Geometry: final body of the model. Coordinates: model frame, mm. A direction names the side the tool comes from. Give positions to 0.01 mm unless a question says otherwise; leave off trailing zeros. Write each loop counter-clockwise with the first axis right and the second up, starting at its lowest first coordinate (ties: lowest second). Pieces come first, ordered by that corner, then holes. Notation, with made-up numbers: (26.5, 38) -> (58.5, 38) arc R25 cw to (58.5, 56) -> close; hole circle Ø2 at (88.5, 35). An arc over 180 degrees is marked (long way). Answer in a Markdown table with one row per item. Add a question column.
Item 1: Section query A-A on y = -13.75. State how many separate pieces and enclosed holes the cut face has, plus the area to 3 significant figures.
Item 2: Access query for faces 1 (the flat face through (15.8, -10.8, 92.1)), 2 (the flat face through (-9.5, -16, 88)), 3 (the flat face through (16.507, 18.048, 38.711)). Directions: +Z, -Z, +X, -X, +Y, -Y. A direction counts if a zero-diameter tool reaches every point of the face in a straight line with its end or side. Return the directions, or none.
Item 3: Draft query along Z for faces 4 (the flat face through (-18.48, -3.58, 29.11)), 5 (the flat face through (13, -18, 12)), 6 (the flat face through (27, 0, 45)). Return one class per face: +Z half, -Z half, draft (parallel to the pull), parting line (faces both ways), or undercut.
Item 4: Material intervals for probe 1 along Y at (x, z) = (13, 4.6); probe 2 along Z at (x, y) = (17.5, -17); probe 3 along Z at (x, y) = (24.25, 13.75), sorted ascending. Write a range as from..to.
Item 5: Section query C-C on x = 22. Output: boundary loops of the cut face in (y, z).
Item 6: Section query D-D on z = 48.5. Output: boundary loops of the cut face in (x, y), plus the area to 3 significant figures.
```python
from build123d import *

# Parameters (mm, degrees)
SKETCH_W            = 54
SKETCH_H            = 44
PAD_DEPTH           = 92.5
SKETCH001_W         = 32
SKETCH001_H         = 44
POCKET_DEPTH        = 86.5
SKETCH002_R         = 2.25
HOLE_DEPTH          = 50
HOLE001_DEPTH       = 50
SKETCH003_R         = 1
HOLE002_DEPTH       = 12
HOLE003_D           = 3.5
HOLE003_DEPTH       = 25
HOLE003_CBORE_D     = 6
HOLE003_CBORE_DEPTH = 6
HOLE003_TIPS_R      = 1.75
POCKET001_DEPTH     = 4
POCKET002_DEPTH     = 4
CHAMFER_SIZE        = 1
SKETCH007_W         = 5
SKETCH007_H         = 8.5
POCKET003_DEPTH     = 13


with BuildPart() as part:
    # Sketch → Pad (new body)
    with BuildSketch(Plane.XY):
        Rectangle(SKETCH_W, SKETCH_H)
    extrude(amount=PAD_DEPTH)

    # Sketch001 (on Face6 of Pad) → Pocket (cut)
    with BuildSketch(Plane.XY.offset(92.5)):
        with Locations((0, 11)):
            Rectangle(SKETCH001_W, SKETCH001_H)
    extrude(amount=-POCKET_DEPTH, mode=Mode.SUBTRACT)

    # Sketch002 → Hole (cut)
    with BuildSketch(Plane.YZ):
        with Locations((0, 41)):
            Circle(SKETCH002_R)
        with Locations((13.75, 41)):
            Circle(SKETCH002_R)
        with Locations((0, 54.75)):
            Circle(SKETCH002_R)
        with Locations((0, 27.25)):
            Circle(SKETCH002_R)
        with Locations((-13.75, 41)):
            Circle(SKETCH002_R)
    extrude(amount=-HOLE_DEPTH, mode=Mode.SUBTRACT)

    # Sketch002 → Hole001 (cut)
    with BuildSketch(Plane.YZ):
        with Locations((0, 41)):
            Circle(SKETCH002_R)
        with Locations((13.75, 41)):
            Circle(SKETCH002_R)
        with Locations((0, 54.75)):
            Circle(SKETCH002_R)
        with Locations((0, 27.25)):
            Circle(SKETCH002_R)
        with Locations((-13.75, 41)):
            Circle(SKETCH002_R)
    extrude(amount=HOLE001_DEPTH, mode=Mode.SUBTRACT)

    # Sketch003 → Hole002 (cut)
    with BuildSketch(Plane.XY):
        with Locations((-13, 18.5)):
            Circle(SKETCH003_R)
        with Locations((13, 18.5)):
            Circle(SKETCH003_R)
        with Locations((13, -18.5)):
            Circle(SKETCH003_R)
        with Locations((-13, -18.5)):
            Circle(SKETCH003_R)
    extrude(amount=HOLE002_DEPTH, mode=Mode.SUBTRACT)

    # Hole003
    with Locations(Plane.XZ.offset(22)):
        with Locations((-11.5, 88), (11.5, 88), (11.5, 55), (-11.5, 55)):
            CounterBoreHole(HOLE003_D / 2, HOLE003_CBORE_D / 2, HOLE003_CBORE_DEPTH, depth=HOLE003_DEPTH)

    # Hole003 tips → Hole003 tip 1 section 0
    with BuildSketch(Plane.XZ.offset(-3), mode=Mode.PRIVATE) as hole003_tip_1_s0:
        with Locations((-11.5, 88)):
            Circle(HOLE003_TIPS_R)
    loft([hole003_tip_1_s0.sketch, Vertex(-11.5, 4.051506, 88)], mode=Mode.SUBTRACT)

    # Hole003 tips → Hole003 tip 2 section 0
    with BuildSketch(Plane.XZ.offset(-3), mode=Mode.PRIVATE) as hole003_tip_2_s0:
        with Locations((11.5, 88)):
            Circle(HOLE003_TIPS_R)
    loft([hole003_tip_2_s0.sketch, Vertex(11.5, 4.051506, 88)], mode=Mode.SUBTRACT)

    # Hole003 tips → Hole003 tip 3 section 0
    with BuildSketch(Plane.XZ.offset(-3), mode=Mode.PRIVATE) as hole003_tip_3_s0:
        with Locations((11.5, 55)):
            Circle(HOLE003_TIPS_R)
    loft([hole003_tip_3_s0.sketch, Vertex(11.5, 4.051506, 55)], mode=Mode.SUBTRACT)

    # Hole003 tips → Hole003 tip 4 section 0
    with BuildSketch(Plane.XZ.offset(-3), mode=Mode.PRIVATE) as hole003_tip_4_s0:
        with Locations((-11.5, 55)):
            Circle(HOLE003_TIPS_R)
    loft([hole003_tip_4_s0.sketch, Vertex(-11.5, 4.051506, 55)], mode=Mode.SUBTRACT)

    # Sketch005 → Pocket001 (cut)
    with BuildSketch(Plane(origin=(16, 0, 0), x_dir=(0, -1, 0), z_dir=(-1, 0, 0))):
        Polygon((2.4, 50.843078), (4.8, 55), (2.4, 59.156922), (-2.4, 59.156922), (-4.8, 55), (-2.4, 50.843078), align=None)
        Polygon((2.4, 36.843078), (4.8, 41), (2.4, 45.156922), (-2.4, 45.156922), (-4.8, 41), (-2.4, 36.843078), align=None)
        Polygon((-11.6, 36.843078), (-9.2, 41), (-11.6, 45.156922), (-16.4, 45.156922), (-18.8, 41), (-16.4, 36.843078), align=None)
        Polygon((2.4, 22.843078), (4.8, 27), (2.4, 31.156922), (-2.4, 31.156922), (-4.8, 27), (-2.4, 22.843078), align=None)
    extrude(amount=-POCKET001_DEPTH, mode=Mode.SUBTRACT)

    # Sketch006 (on Face7 of Hole003) → Pocket002 (cut)
    with BuildSketch(Plane.YZ.offset(-16)):
        Polygon((2.4, 50.843078), (4.8, 55), (2.4, 59.156922), (-2.4, 59.156922), (-4.8, 55), (-2.4, 50.843078), align=None)
        Polygon((2.4, 36.843078), (4.8, 41), (2.4, 45.156922), (-2.4, 45.156922), (-4.8, 41), (-2.4, 36.843078), align=None)
        Polygon((16.4, 36.843078), (18.8, 41), (16.4, 45.156922), (11.6, 45.156922), (9.2, 41), (11.6, 36.843078), align=None)
        Polygon((2.4, 22.843078), (4.8, 27), (2.4, 31.156922), (-2.4, 31.156922), (-4.8, 27), (-2.4, 22.843078), align=None)
    extrude(amount=-POCKET002_DEPTH, mode=Mode.SUBTRACT)

    # Chamfer
    chamfer_edges = [part.edges().sort_by_distance(p)[0] for p in [
        (-27, 22, 46.25),
        (-27, -22, 46.25),
        (27, 22, 46.25),
        (27, -22, 46.25),
        (27, 0, 92.5),
        (16, 5.5, 92.5),
        (0, -11, 92.5),
        (-16, 5.5, 92.5),
        (0, -22, 92.5),
        (-27, 0, 92.5),
        (-21.5, 22, 92.5),
        (21.5, 22, 92.5),
        (16, 22, 49.25),
        (0, 22, 6),
        (-16, 22, 49.25),
        (-16, 3.6, 57.078461),
        (-16, 0, 59.156922),
        (-16, -3.6, 57.078461),
        (-16, -3.6, 52.921539),
        (-16, 0, 50.843078),
        (-16, 3.6, 52.921539),
        (-16, 0, 45.156922),
        (-16, -3.6, 43.078461),
        (-16, -3.6, 38.921539),
        (-16, 0, 36.843078),
        (-16, 3.6, 38.921539),
        (-16, 3.6, 43.078461),
        (-16, 14, 45.156922),
        (-16, 10.4, 43.078461),
        (-16, 10.4, 38.921539),
        (-16, 14, 36.843078),
        (-16, 17.6, 38.921539),
        (-16, 17.6, 43.078461),
        (-16, 0, 31.156922),
        (-16, -3.6, 29.078461),
        (-16, -3.6, 24.921539),
        (-16, 0, 22.843078),
        (-16, 3.6, 24.921539),
        (-16, 3.6, 29.078461),
        (16, -3.6, 57.078461),
        (16, 0, 59.156922),
        (16, 3.6, 57.078461),
        (16, 3.6, 52.921539),
        (16, 0, 50.843078),
        (16, -3.6, 52.921539),
        (16, 0, 45.156922),
        (16, -3.6, 43.078461),
        (16, -3.6, 38.921539),
        (16, 0, 36.843078),
        (16, -11, 49.25),
        (16, 5.5, 6),
        (16, -3.6, 24.921539),
        (16, -3.6, 29.078461),
        (16, 0, 31.156922),
        (16, 3.6, 29.078461),
        (16, 3.6, 24.921539),
        (16, 0, 22.843078),
        (16, 10.4, 38.921539),
        (16, 10.4, 43.078461),
        (16, 14, 45.156922),
        (16, 17.6, 43.078461),
        (16, 17.6, 38.921539),
        (16, 14, 36.843078),
        (16, 3.6, 43.078461),
        (16, 3.6, 38.921539),
    ]]
    chamfer(chamfer_edges, length=CHAMFER_SIZE)

    # Sketch007 (on Face15 of Chamfer) → Pocket003 (cut)
    with BuildSketch(Plane.XZ.offset(22)):
        with Locations((-17.5, 41)):
            Rectangle(SKETCH007_W, SKETCH007_H)
        with Locations((17.5, 41)):
            Rectangle(SKETCH007_W, SKETCH007_H)
    extrude(amount=-POCKET003_DEPTH, mode=Mode.SUBTRACT)


solid = part.part
```
Findings below:
| question | item | result |
|---|---|---|
| 1 | separate pieces | 2 |
| 1 | enclosed holes | 4 |
| 1 | area | 4,670 mm^2 |
| 2 | face 1 | +Z, +Y |
| 2 | face 2 | -Y |
| 2 | face 3 | none |
| 3 | face 4 | undercut |
| 3 | face 5 | -Z half |
| 3 | face 6 | draft |
| 4 | probe 1 | y = -22..-19.5, -17.5..17.5, 19.5..22 |
| 4 | probe 2 | z = 0..36.75, 45.25..92.5 |
| 4 | probe 3 | z = 0..38.75, 43.25..92.5 |
| 5 | outline | (-22, 0) -> (22, 0) -> (22, 91.5) -> (21, 92.5) -> (-21, 92.5) -> (-22, 91.5) -> close; hole circle Ø4.5 at (-13.75, 41); hole circle Ø4.5 at (0, 27.25); hole circle Ø4.5 at (0, 41); hole circle Ø4.5 at (0, 54.75); hole circle Ø4.5 at (13.75, 41) |
| 6 | outline | (-27, -21) -> (-26, -22) -> (26, -22) -> (27, -21) -> (27, 21) -> (26, 22) -> (17, 22) -> (16, 21) -> (16, -10) -> (15, -11) -> (-16, -11) -> (-16, 21) -> (-17, 22) -> (-26, 22) -> (-27, 21) -> close |
| 6 | area | 1,320 mm^2 |
